Can you work these out from the model? Positions are in its coordinate system, mm. A direction names the side the tool comes from. Round coordinates to 2 decimals unless told otherwise and drop trailing zeros. Loops run counter-clockwise (first coordinate to the right, second up) from the corner with the lowest first, then second, coordinate; pieces in that order, holes last. Notation, with made-up numbers: (29, 8) - (84, 8) arc R19 ccw to (84, 29) - close; hole circle Ø2 at (-31, -4.5). An arc over 180 degrees is marked (long way). Answer as CSV lines item,"result".
Autodesk Inventor part; units mm, degrees
ref_plane "YZ Plane" through (0, 0, 0) normal (1, 0, 0) x (0, 1, 0)
ref_plane "XZ Plane" through (0, 0, 0) normal (0, 1, 0) x (-1, 0, 0)
ref_plane "XY Plane" through (0, 0, 0) normal (0, 0, 1) x (1, 0, 0)
sketch "Sketch1" plane through (0, 0, 0) normal (0, 1, 0) x (-1, 0, 0)
  line L0 (26, 0) -> (0, 0)
  line L1 (0, 0) -> (0, -38)
  line L2 (0, -38) -> (26, -38)
  line L3 (26, -38) -> (26, 0)
  dimension "d0" = 38
  dimension "d1" = 26
extrude "Extrusion1" add sketch "Sketch1" along normal blind 21
sketch "Sketch2" plane through (0, 21, 0) normal (0, 1, 0) x (1, 0, 0)
  line L0 (-19.5, 30) -> (-6.5, 30)
  line L1 (0, 38) -> (-26, 38)
  line L2 (-26, 38) -> (-26, 0)
  line L3 (-6.5, 30) -> (-6.5, 23)
  line L4 (-13, 30) -> (-13, 10.7779) construction
  line L5 (-16.5, 21) -> (-9.5, 21)
  line L6 (-6.5, 23) -> (-9.5, 23)
  line L7 (-9.5, 23) -> (-9.5, 21)
  line L8 (-16.5, 21) -> (-16.5, 23)
  line L9 (-16.5, 23) -> (-19.5, 23)
  line L10 (-19.5, 23) -> (-19.5, 30)
  point P0 (0, 0)
  point P1 (-13, 21)
  point P2 (-13, 26.5)
  dimension "d4" = 8
  dimension "d5" = 13
  dimension "d6" = 26
  dimension "d7" = 6.5
  dimension "d8" = 7
  dimension "d9" = 7
  dimension "d10" = 2
extrude "Extrusion2" cut sketch "Sketch2" against normal blind 15
sketch "Sketch3" plane through (-26, 0, 0) normal (0, 0, 1) x (1, 0, 0)
  line L0 (5.5, 5) -> (20.5, 5)
  line L1 (0, 0) -> (26, 0)
  line L2 (13, 0) -> (13, 33.23) construction
  line L3 (5.5, 5) -> (5.5, 12)
  line L4 (5.5, 12) -> (20.5, 12)
  line L5 (20.5, 12) -> (20.5, 5)
  line L6 (6, 11.5) -> (20, 11.5)
  line L7 (20, 11.5) -> (20, 8.5)
  line L8 (20, 8.5) -> (6, 8.5)
  line L9 (6, 8.5) -> (6, 11.5)
  point P0 (13, 5)
  point P1 (13, 8.5)
  dimension "d13" = 5
  dimension "d14" = 15
  dimension "d15" = 7
  dimension "d16" = 14
  dimension "d17" = 3
  dimension "d18" = 0.5
  dimension "d19" = 0.5
extrude "Extrusion3" cut sketch "Sketch3" against normal blind 15
equation "\"d7\" = -0.5 * d5 + 0.5 * d6"
properties part number "usbRangeExtender"
Q1. Imagine slicing it at B-B (z = -6). Write out the boundary of the cut face in (x, y).
Checks:
outline,"(-26, 0) - (0, 0) - (0, 21) - (-26, 21) - close; (-20, 8.5) - (-6, 8.5) - (-6, 11.5) - (-20, 11.5) - close; hole (-20.5, 5) - (-5.5, 5) - (-5.5, 12) - (-20.5, 12) - close"
Q2. On a 3-axis mill with a long thin cutter (end or side, diameter ignored), from which of +Z, -Z, +X, -X, +Y, -Y can I reach the whole of each face in a straight line? I mean faces 1 (the flat face through (-13, 14, -30)), 2 (the flat face through (-20.5, 8, -7)), 3 (the flat face through (-13, 0, -19)). Say none if no direction works.
Checks:
face 1,"+Y"
face 2,"+Z"
face 3,"+Z, -Z, +X, -X, -Y"
Q3. I'm going to push flat-ended pins straight in: pin 1 Ø2 at (y, z) = (11, -26) entering from +X; pin 2 Ø2.5 at (x, z) = (-13, -26.5) entering from +Y; pin 3 Ø1.5 at (x, y) = (-15, 6.5) entering from +Z. Where does each tip first touch, or does it pass through?
Checks:
pin 1,"x = 0"
pin 2,"y = 6"
pin 3,"z = -15"
Q4. Imagine slicing it at A-A (y = 14.25). Write out the boundary of the cut face in (x, z), then the cut area to 3 significant figures.
Checks:
outline,"(-26, -38) - (0, -38) - (0, 0) - (-26, 0) - close; hole (-19.5, -30) - (-6.5, -30) - (-6.5, -23) - (-9.5, -23) - (-9.5, -21) - (-16.5, -21) - (-16.5, -23) - (-19.5, -23) - close"
area,"883 mm²"
Q5. We'd pull the mould along X, two halves only. Please class faces 4 (the flat face through (-13, 10, 0)), 5 (the flat face through (0, 10, -19)), 6 (the flat face through (-13, 12, -7)): pulls with the +X half, pulls with the -X half, needs draft (parallel to the pull), parting line crosses it, or undercut.
Checks:
face 4,"needs draft"
face 5,"pulls with the +X half"
face 6,"undercut"
Q6. If I drill on line 1 along Y through (x, z) = (-19.75, -13); line 2 along X through (y, z) = (15.25, -27); line 3 along Z through (x, y) = (-8.75, 19), over which ranges is the centre line in solid material (lowest first)? Write a range as [from, to].
Checks:
line 1,"[0, 5], [8.5, 11.5], [12, 21]"
line 2,"[-26, -19.5], [-6.5, 0]"
line 3,"[-38, -30], [-23, 0]"
Q7. Imagine slicing it at D-D (z = -28). Write out the boundary of the cut face in (x, y).
Checks:
outline,"(-26, 0) - (0, 0) - (0, 21) - (-6.5, 21) - (-6.5, 6) - (-19.5, 6) - (-19.5, 21) - (-26, 21) - close"
Q8. Imagine slicing it at C-C (x = -13.5). Write out the boundary of the cut face in (y, z), then the cut area to 3 significant figures.
Checks:
outline,"(0, -38) - (21, -38) - (21, -30) - (6, -30) - (6, -21) - (21, -21) - (21, 0) - (12, 0) - (12, -15) - (11.5, -15) - (11.5, 0) - (8.5, 0) - (8.5, -15) - (5, -15) - (5, 0) - (0, 0) - close"
area,"603 mm²"
